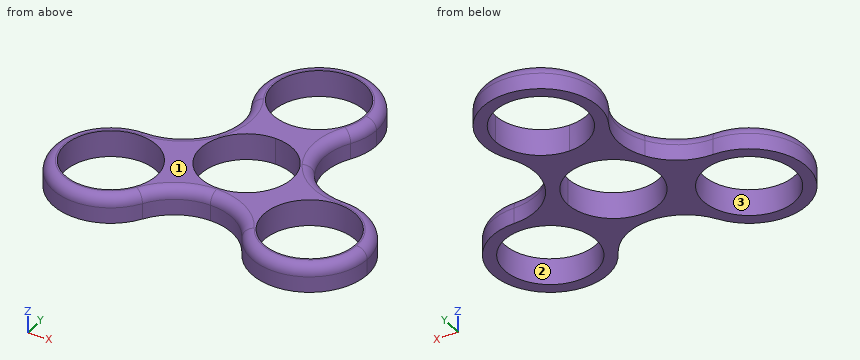
from build123d import *

# Parameters (mm, degrees)
F0_R     = 11.049
F1_DEPTH = 6.35
F2_R     = 2.54


# Not quite as in the source:
# - ends of sketch curves that miss each other by under 0.0002 mm in the source are joined


with BuildPart() as f1:
    # F0 (on Top) → F1 (new body)
    with BuildSketch(Plane.XY):
        with BuildLine():
            ThreePointArc((0, 11.049), (7.8128228253, 7.8128228253), (11.049, 0))
            ThreePointArc((11.049, 0), (-2.8596916293, -10.6725144547), (-9.5687146864, 5.5245))
            Line((-9.5687146864, 5.5245), (-12.0983748909, 6.985))
            ThreePointArc((-12.0983748909, 6.985), (-13.97, 3.443e-07), (-12.0983754224, -6.9849990793))
            ThreePointArc((-12.0983754224, -6.9849990793), (-6.9850004566, -12.0983746273), (8.7e-09, -13.97))
            ThreePointArc((8.7e-09, -13.97), (6.9850004798, -12.0983746139), (12.0983754405, -6.984999048))
            ThreePointArc((12.0983754405, -6.984999048), (13.4939839355, -3.6157015292), (13.97, 0))
            ThreePointArc((13.97, 0), (13.4939839355, 3.6157015292), (12.0983754405, 6.984999048))
            ThreePointArc((12.0983754405, 6.984999048), (6.9850004648, 12.0983746225), (-2.58e-08, 13.97))
            Line((-2.58e-08, 13.97), (0, 11.049))
        make_face()
        with BuildLine():
            ThreePointArc((-9.5687146864, 5.5245), (-5.5245, 9.5687146864), (0, 11.049))
            Line((0, 11.049), (0, 13.97))
            ThreePointArc((0, 13.97), (-6.9850001734, 12.0983747908), (-12.0983750781, 6.9849996757))
            Line((-12.0983750781, 6.9849996757), (-9.5687146864, 5.5245))
        make_face()
        with BuildLine():
            ThreePointArc((-12.0983750781, 6.9849996757), (-6.9850001734, 12.0983747908), (-2.58e-08, 13.97))
            ThreePointArc((-2.58e-08, 13.97), (-6.9850000112, 15.8416251156), (-12.0983748909, 20.955))
            ThreePointArc((-12.0983748909, 20.955), (-10.2267497817, 13.9699998127), (-12.0983750781, 6.9849996757))
        make_face()
        with BuildLine():
            ThreePointArc((-12.0983748909, 20.955), (-6.9850000112, 15.8416251156), (-2.58e-08, 13.97))
            ThreePointArc((-2.58e-08, 13.97), (6.9849999888, 15.8416251027), (12.0983748909, 20.955))
            ThreePointArc((12.0983748909, 20.955), (13.4939837933, 24.3242979399), (13.97, 27.94))
            ThreePointArc((13.97, 27.94), (-3.6157020601, 41.4339837933), (-12.0983748909, 20.955))
        make_face()
        with BuildLine():
            ThreePointArc((11.049, 27.94), (7.8128228253, 20.1271771747), (0, 16.891))
            ThreePointArc((0, 16.891), (-7.8128228253, 35.7528228253), (11.049, 27.94))
        make_face(mode=Mode.SUBTRACT)
        with BuildLine():
            ThreePointArc((12.0983748909, 20.955), (6.9849999888, 15.8416251027), (-2.58e-08, 13.97))
            ThreePointArc((-2.58e-08, 13.97), (6.9850004648, 12.0983746225), (12.0983754405, 6.984999048))
            ThreePointArc((12.0983754405, 6.984999048), (10.2267497817, 13.9699994504), (12.0983748909, 20.955))
        make_face()
        with BuildLine():
            ThreePointArc((-12.0983754224, -6.9849990793), (-13.97, 3.443e-07), (-12.0983750781, 6.9849996757))
            ThreePointArc((-12.0983750781, 6.9849996757), (-17.2117499439, 1.8716250155), (-24.1967497817, 0))
            ThreePointArc((-24.1967497817, 0), (-17.2117502421, -1.8716248433), (-12.0983754224, -6.9849990793))
        make_face()
        with BuildLine():
            ThreePointArc((24.1967497817, 0), (17.2117502577, 1.8716248343), (12.0983754405, 6.984999048))
            ThreePointArc((12.0983754405, 6.984999048), (13.4939839355, 3.6157015292), (13.97, 0))
            ThreePointArc((13.97, 0), (13.4939839355, -3.6157015292), (12.0983754405, -6.984999048))
            ThreePointArc((12.0983754405, -6.984999048), (17.2117502577, -1.8716248343), (24.1967497817, 0))
        make_face()
        with BuildLine():
            ThreePointArc((8.7e-09, -13.97), (-6.9850004566, -12.0983746273), (-12.0983754224, -6.9849990793))
            ThreePointArc((-12.0983754224, -6.9849990793), (-10.7027661261, -10.3542974265), (-10.2267497817, -13.97))
            ThreePointArc((-10.2267497817, -13.97), (-10.7027659885, -17.5857020601), (-12.0983748909, -20.955))
            ThreePointArc((-12.0983748909, -20.955), (-6.9849999962, -15.841625107), (8.7e-09, -13.97))
        make_face()
        with BuildLine():
            ThreePointArc((-10.2267497817, -13.97), (-10.7027661261, -10.3542974265), (-12.0983754224, -6.9849990793))
            ThreePointArc((-12.0983754224, -6.9849990793), (-17.2117502421, -1.8716248433), (-24.1967497817, 0))
            ThreePointArc((-24.1967497817, 0), (-36.2951246726, -20.955), (-12.0983748909, -20.955))
            ThreePointArc((-12.0983748909, -20.955), (-10.7027659885, -17.5857020601), (-10.2267497817, -13.97))
        make_face()
        with Locations((-24.1967497817, -13.97)):
            Circle(F0_R, mode=Mode.SUBTRACT)
        with BuildLine():
            ThreePointArc((38.1667497817, -13.97), (34.0750315149, -4.0917182668), (24.1967497817, 0))
            ThreePointArc((24.1967497817, 0), (17.2117502577, -1.8716248343), (12.0983754405, -6.984999048))
            ThreePointArc((12.0983754405, -6.984999048), (10.2267497817, -13.9699994504), (12.0983748909, -20.955))
            ThreePointArc((12.0983748909, -20.955), (27.8124518418, -27.4639837933), (38.1667497817, -13.97))
        make_face()
        with Locations((24.1967497817, -13.97)):
            Circle(F0_R, mode=Mode.SUBTRACT)
        with BuildLine():
            ThreePointArc((12.0983754405, -6.984999048), (6.9850004798, -12.0983746139), (8.7e-09, -13.97))
            ThreePointArc((8.7e-09, -13.97), (6.9850000038, -15.8416251113), (12.0983748909, -20.955))
            ThreePointArc((12.0983748909, -20.955), (10.2267497817, -13.9699994504), (12.0983754405, -6.984999048))
        make_face()
    extrude(amount=F1_DEPTH)

    # F2
    f2_edges = [f1.edges().sort_by_distance(p)[0] for p in [
        (0, -13.97, 6.35),
        (36.295125, -20.955, 6.35),
        (12.098375, 6.985, 6.35),
        (0, 41.91, 6.35),
        (-12.098375, 6.985, 6.35),
        (-36.295125, -20.955, 6.35),
    ]]
    fillet(f2_edges, radius=F2_R)


solid = f1.part
Could you check a few things on this model? Use its own coordinates, in mm. Face numbers are marked on the shaded views. Give positions to 0.01 mm unless a question says otherwise; leave off trailing zeros. Order: outer loops, then holes, each group sorted by start corner. A loop starts at its lowest first (then second) coordinate and runs counter-clockwise, first axis right, second up. Notation, with made-up numbers: (59.25, 87) - (87.25, 87) arc R19 cw to (87.25, 99) - close; hole circle Ø2 at (56, -33). An arc over 180 degrees is marked (long way). One line per item, written item: value. Start each with the question number.
1. For P1, Ø2, axis at x = 19, z = 5.5, coming from the -Y side; P2, Ø2, axis at y = -21, z = 3.5, coming from the -X side; P3, Ø3, axis at x = 6.5, z = 5.5, coming from the +Y side, each with a flat end and sliding along its axis, tell me the tip position at first contact or that it passes through.
2. Imagine slicing it at A-A on z = 2. List the corners of the cut face in (x, y) for me (3 decimals).
3. If I drill on probe 1 along X at (y, z) = (-13, 3.75); probe 2 along X at (y, z) = (-21, 2.75); probe 3 along X at (y, z) = (-9, 5.75), over which ranges is the centre line in solid material (lowest first)?
4. Thinking about a two-plate mould opening in Y: for the marked faces 1, 2 and 3, which applies, +Y half, -Y half, draft (parallel to the pull), parting line (faces both ways), or undercut?
Values:
1. P1: y = -26.99
1. P2: x = -36.8
1. P3: y = 40.73
2. outline: (-24.197, 0) arc R13.97 ccw (long way) to (-12.098, -20.955) arc R13.97 cw to (12.098, -20.955) arc R13.97 ccw (long way) to (24.197, 0) arc R13.97 cw to (12.098, 20.955) arc R13.97 ccw (long way) to (-12.098, 20.955) arc R13.97 cw to start; hole circle Ø22.098 at (-24.197, -13.97); hole circle Ø22.098 at (0, 0); hole circle Ø22.098 at (0, 27.94); hole circle Ø22.098 at (24.197, -13.97)
3. probe 1: -38.13 to -35.2, -13.19 to 13.19, 35.2 to 38.13
3. probe 2: -36.27 to -32.72, -15.67 to -12.12, 12.12 to 15.67, 32.72 to 36.27
3. probe 3: -36.28 to -34.06, -14.33 to -6.41, 6.41 to 14.33, 34.06 to 36.28
4. face 1: draft
4. face 2: undercut
4. face 3: undercut
